Input: part model. Units: mm. Frame: model coordinates. A direction names the side the tool comes from. Round coordinates to 2 decimals unless told otherwise and drop trailing zeros. Order: outer loops, then holes, each group sorted by start corner. A loop starts at its lowest first (then second) coordinate and runs counter-clockwise, first axis right, second up.
Item 1: Cut plane C-C on y = 8.5. Output: boundary loops of the cut face in (x, z) (3 decimals), then the cut area to 3 significant figures.
Item 2: First-contact query: pin 1 (2 mm diameter, centred on x = 10, z = 1.5, fed in from +Y); pin 2 (2 mm diameter, centred on x = 5, z = -31, fed in from -Y); pin 3 (2 mm diameter, centred on x = 12, y = 18.5, fed in from -Z). Flat tips, straight axial feed; report the tip coordinate or a pass-through.
Item 3: Reachability of faces 4 (the cylindrical face through (-2.41, 61.65, -31.84)), 5 (the flat face through (5, 63, -50.8)), 6 (the flat face through (0.88, 12.7, -11.23)) from +Z, -Z, +X, -X, +Y, -Y: full face, straight path, thin tool, end or side. Return the list, or none.
Item 4: Line query: L1, parallel to Y at x = 0, z = -32.5 (1 decimal); L2, parallel to Y at x = 0, z = -42 (3 decimals); L3, parallel to X at y = 50.8, z = -35.5 (1 decimal). Output: solid intervals per line, ascending.
Item 5: Mould query, pull axis X, two halves, no side actions, for faces 1 (the cylindrical face through (-3.441, 12.878, 15.497)), 2 (the flat face through (11, 0, 7)), 3 (the cylindrical face through (10.6, 19.14, -3.34)). Classes: released by +X, released by -X, zero draft, split by the parting line, or undercut.
```python
from build123d import *

# Parameters (mm, degrees)
F0_R     = 15.875
F0_R_2   = 11.1125
F3_R     = 12.7
F3_R_2   = 11.1125
F4_DEPTH = 12.7
F5_R     = 12.7
F5_R_2   = 11.1125
F6_DEPTH = 12.7


with BuildPart() as f2:
    # F2: sweep along a path in F1
    with BuildLine(Plane.YZ) as f2_path:
        Line((0, 0), (25.4, 0))
        ThreePointArc((25.4, 0), (43.3605122421, -7.4394877579), (50.8, -25.4))
        Line((50.8, -25.4), (50.8, -50.8))
    # F0 (on Front) → F2 (sweep)
    with BuildSketch(Plane.XZ):
        Circle(F0_R)
        Circle(F0_R_2, mode=Mode.SUBTRACT)
    sweep(path=f2_path.line)

    # F3 (on face) → F4 (cut)
    with BuildSketch(Plane.XZ):
        Circle(F3_R)
        Circle(F3_R_2, mode=Mode.SUBTRACT)
    extrude(amount=-F4_DEPTH, mode=Mode.SUBTRACT)

    # F5 (on face) → F6 (cut)
    with BuildSketch(Plane(origin=(0, 0, -50.8), x_dir=(1, 0, 0), z_dir=(0, 0, -1))):
        with Locations((0, -50.8)):
            Circle(F5_R)
        with Locations((0, -50.8)):
            Circle(F5_R_2, mode=Mode.SUBTRACT)
    extrude(amount=-F6_DEPTH, mode=Mode.SUBTRACT)


solid = f2.part
```
From the geometry:
1. outline: circle Ø31.75 at (0, 0); hole circle Ø25.4 at (0, 0)
1. area: 285 mm2
2. pin 1: stops at y = 53.3
2. pin 2: stops at y = 35.44
2. pin 3: stops at z = -11.45
3. face 4: -Z
3. face 5: -Z, +X, -X, +Y, -Y
3. face 6: -Y
4. L1: y = 34.9 to 39.7, 61.9 to 66.7
4. L2: y = 34.925 to 38.1, 63.5 to 66.675
4. L3: x = -15.9 to -11.1, 11.1 to 15.9
5. face 1: split by the parting line
5. face 2: zero draft
5. face 3: undercut
